Part model, mm, in its own coordinate system. A direction names the side the tool comes from. Give positions to 0.01 mm unless a question says otherwise; leave off trailing zeros. Order: outer loops, then holes, each group sorted by start corner. A loop starts at its lowest first (then second) coordinate and runs counter-clockwise, first axis right, second up.
from build123d import *

# Parameters (mm, degrees)
F0_R     = 6.25
F3_R     = 5.5
F5_DEPTH = 65
F1_R     = 3.25
F6_DEPTH = 65


with BuildPart() as f4:
    # F0 (on Top) → F4 section 0
    with BuildSketch(Plane.XY):
        Circle(F0_R)
    # F3 (on offset) → F4 section 1
    with BuildSketch(Plane.XY.offset(-7.5)):
        Circle(F3_R)
    loft()

    # F0 (on Top) → F5 (join)
    with BuildSketch(Plane.XY):
        Circle(F0_R)
    extrude(amount=F5_DEPTH)

    # F1 (on Top) → F6 (cut)
    with BuildSketch(Plane.XY):
        Circle(F1_R)
    extrude(amount=F6_DEPTH, mode=Mode.SUBTRACT)


solid = f4.part
Item 1: Drill centre lines: probe 1 along Y at (x, z) = (0, 13); probe 2 along X at (y, z) = (-0.25, 43) (3 decimals); probe 3 along Z at (x, y) = (-2.25, 0.25). Where is each one in solid material? Low to high.
Item 2: Pull direction X, two halves, no side cores. Call faces 1 (the face through (-2.579, -1.978, 32.045)), 2 (the face through (3, -3, 65)), 3 (the face through (5.96, 1.88, 32.04)): released by +X, released by -X, zero draft, split by the parting line, or undercut.
Item 3: Band-saw the part on A-A on x = 0. List the corners of the cut face in (y, z), plus the area to 3 significant figures.
Item 4: Which spindle directions (+Z, -Z, +X, -X, +Y, -Y) get a long thin tool onto all of the face, cutting with end or side? Do faces 4 (the face through (0, 0, 0)), 5 (the face through (0, 0, -7.5)). Say none if no direction does.
Item 5: Band-saw the part on B-B on z = 14. List the corners of the cut face in (x, y), plus the area to 3 significant figures.
Item 6: Drop flat-ended pins along their axis: P1, Ø3, axis at x = 0, y = 1.5, coming from the +Z side; P2, Ø1.5, axis at x = -2, z = 0, coming from the +Y side. Give the stop position or say it passes through.
Working result:
1. probe 1: y = -6.25 to -3.25, 3.25 to 6.25
1. probe 2: x = -6.245 to -3.24, 3.24 to 6.245
1. probe 3: z = -7.5 to 0
2. face 1: undercut
2. face 2: zero draft
2. face 3: split by the parting line
3. outline: (-6.25, 0) - (-5.5, -7.5) - (5.5, -7.5) - (6.25, 0) - (6.25, 65) - (3.25, 65) - (3.25, 0) - (-3.25, 0) - (-3.25, 65) - (-6.25, 65) - close
3. area: 478 mm2
4. face 4: +Z
4. face 5: -Z, +X, -X, +Y, -Y
5. outline: circle Ø12.5 at (0, 0); hole circle Ø6.5 at (0, 0)
5. area: 89.5 mm2
6. P1: stops at z = 0
6. P2: stops at y = 6.12
